from build123d import *

# Parameters (mm, degrees)
F0_W           = 35
F0_H           = 100
F1_DEPTH       = 40
F2_W           = 27.5
F2_H           = 90
F3_DEPTH       = 26
F4_R           = 10
F6_D           = 8.5
F6_CBORE_D     = 20
F6_CBORE_DEPTH = 8


with BuildPart() as f1:
    # F0 (on Front) → F1 (new body)
    with BuildSketch(Plane.XZ):
        Rectangle(F0_W, F0_H)
    extrude(amount=F1_DEPTH)

    # F2 (on face) → F3 (cut)
    with BuildSketch(Plane.XZ.offset(40)):
        with Locations((0, 5)):
            Rectangle(F2_W, F2_H)
    extrude(amount=-F3_DEPTH, mode=Mode.SUBTRACT)

    # F4
    f4_edges = [f1.edges().sort_by_distance(p)[0] for p in [
        (-15.625, -40, 50),
        (15.625, -40, 50),
        (-17.5, -20, -50),
        (17.5, -20, -50),
    ]]
    fillet(f4_edges, radius=F4_R)

    # F6 (through all)
    with Locations(Plane.XZ.offset(14)):
        with Locations((0, 30), (0, -30)):
            CounterBoreHole(F6_D / 2, F6_CBORE_D / 2, F6_CBORE_DEPTH)


solid = f1.part
Build history of the part. All positions in model axes, mm. A direction names the side the tool comes from. Coordinates: 2 decimals unless noted, no trailing zeros. Order: outer loops, then holes, each group sorted by start corner. A loop starts at its lowest first (then second) coordinate and runs counter-clockwise, first axis right, second up. Notation, with made-up numbers: (31.25, 45) - (64.25, 45) arc R10 ccw to (64.25, 61) - close; hole circle Ø8 at (70.5, -2). An arc over 180 degrees is marked (long way). Write each question's results on one line, items separated by ' | '. Start each with the question number.
Item 1: Tool access for faces 1 (the face through (0.92, -2.96, 25.85)), 2 (the face through (2, -6, -34)), 3 (the face through (0, -14, 6)): list every direction of +Z, -Z, +X, -X, +Y, -Y with a clear straight run to the whole face (end or side of a thin tool).
Item 2: Band-saw the part on C-C on z = -1.5. Write the cut outline in (x, y), and give its area (3 significant figures).
Item 3: Flat gauge pins, fed straight in: pin 1 (1 mm diameter, centred on x = 5.5, z = -38.5, fed in from -Y); pin 2 (12 mm diameter, centred on x = 0, z = 30, fed in from -Y); pin 3 (5 mm diameter, centred on x = 4, y = -25.5, fed in from +Z). Where does each tip first touch, or does it go through?
Item 4: Mould opens along Z. For faces 4 (the face through (-17.5, -20, 4)), 5 (the face through (4, -6, 28)), 6 (the face through (-14.65, -20.28, -46.99)) say: released by +Z, released by -Z, zero draft, split by the parting line, or undercut.
Item 5: Band-saw the part on D-D on y = -17. Write the cut outline in (x, z).
Item 6: Band-saw the part on A-A on z = -30. Write the cut outline in (x, y), and give its area (3 significant figures).
Item 7: Wall check: probe 1 along Z at (x, y) = (0, -4); probe 2 along Z at (x, y) = (0, -10.25); probe 3 along X at (y, z) = (-20.5, -14). Give the ranges that are in metal, low to high. Write a range as [from, to].
Item 8: Band-saw the part on B-B on y = -11.5. Write the cut outline in (x, z).
Numbers:
1) face 1: +Y, -Y | face 2: -Y | face 3: +Z, -Y
2) outline: (-17.5, -40) - (-13.75, -40) - (-13.75, -14) - (13.75, -14) - (13.75, -40) - (17.5, -40) - (17.5, 0) - (-17.5, 0) - close | area: 685 mm^2
3) pin 1: y = -14 | pin 2: y = -6 | pin 3: z = -40
4) face 4: zero draft | face 5: undercut | face 6: released by -Z
5) outline: (-17.5, -40) arc R10 ccw to (-7.5, -50) - (7.5, -50) arc R10 ccw to (17.5, -40) - (17.5, 50) - (13.75, 50) - (13.75, -40) - (-13.75, -40) - (-13.75, 50) - (-17.5, 50) - close
6) outline: (-17.5, -40) - (-13.75, -40) - (-13.75, -14) - (-10, -14) - (-10, -6) - (-4.25, -6) - (-4.25, 0) - (-17.5, 0) - close; (4.25, -6) - (10, -6) - (10, -14) - (13.75, -14) - (13.75, -40) - (17.5, -40) - (17.5, 0) - (4.25, 0) - close | area: 474 mm^2
7) probe 1: [-50, -34.25], [-25.75, 25.75], [34.25, 50] | probe 2: [-50, -40], [-20, 20], [40, 50] | probe 3: [-17.5, -13.75], [13.75, 17.5]
8) outline: (-17.5, -40) arc R10 ccw to (-7.5, -50) - (7.5, -50) arc R10 ccw to (17.5, -40) - (17.5, 50) - (-17.5, 50) - close; hole circle Ø20 at (0, -30); hole circle Ø20 at (0, 30)
